Autodesk Inventor part; units mm, degrees
ref_plane "YZ-Ebene" through (0, 0, 0) normal (1, 0, 0) x (0, 1, 0)
ref_plane "XZ-Ebene" through (0, 0, 0) normal (0, 1, 0) x (-1, 0, 0)
sketch "Skizze1" plane through (0, 0, 0) normal (0, 0, 1) x (1, 0, 0)
  line L0 (-14.4, 0) -> (2.4, 0)
  line L1 (0, -0.9) -> (0, 5.4)
  line L2 (-12, 1.7) -> (-12, 2)
  line L3 (-12, 2) -> (-11, 2)
  line L4 (-11, 2) -> (-11, 4.5)
  line L5 (-11, 4.5) -> (0, 4.5)
  line L6 (-12, 1.7) -> (0, 1.7)
  line L7 (0, 4.5) -> (0, 1.7)
  point P0 (0, 0)
  dimension "d1" = 3.4
  dimension "d2" = 4
  dimension "d3" = 11
  dimension "d4" = 12
  dimension "d5" = 9
revolve "Umdrehung1" add sketch "Skizze1" angle 360 about axis through (-10, 0, 0) along (1, 0, 0)
ref_plane "Arbeitsebene1" through (-5.5, 0, 4.5) normal (0, 0, 1) x (1, 0, 0)
sketch "Skizze2" plane through (-5.5, 0, 4.5) normal (0, 0, 1) x (1, 0, 0)
  line L0 (-5.5, 4.5) -> (5.5, 4.5)
  line L1 (5.5, -4.5) -> (5.5, 4.5)
  line L2 (3, 4.5) -> (5.5, 4.5)
  line L3 (5.5, 4.5) -> (5.5, 2.6)
  line L4 (5.5, 2.6) -> (3, 2.6)
  line L5 (3, 2.6) -> (3, 4.5)
  point P0 (5.5, 0)
  dimension "d9" = 1.9
  dimension "d10" = 2.5
extrude "Extrusion1" cut sketch "Skizze2" against normal through all
ref_plane "Arbeitsebene2" through (-5.5, 0, 4.5) normal (0, 0, 1) x (1, 0, 0)
sketch "Skizze3" plane through (-5.5, 0, 4.5) normal (0, 0, 1) x (1, 0, 0)
  line L0 (-8.9, 0) -> (7.9, 0)
  line L1 (-5.5, -4.5) -> (-5.5, 4.5)
  line L2 (5.5, -4.5) -> (5.5, 2.6)
  circle A0 centre (0, 0) radius 2.25
  point P0 (5.5, 0)
  dimension "d13" = 4.5
  dimension "d14" = 5.5
extrude "Extrusion2" cut sketch "Skizze3" against normal through all
properties part number "Schließbahn_ra8846s" material "Stahl"
For this review, take the finished solid that the model builds, in its own axes (mm). A direction names the side the tool comes from. Round coordinates to 2 decimals unless told otherwise and drop trailing zeros. Write each loop counter-clockwise with the first axis right and the second up, starting at its lowest first coordinate (ties: lowest second). Pieces come first, ordered by that corner, then holes.
1) For line 1 along Z through (x, y) = (-8.1, 0); line 2 along X through (y, z) = (3.5, -1.75), list the stretches that pass through material, from the lowest coordinate up.
Answer below:
line 1: z = -4.5 to -1.7, 1.7 to 4.5
line 2: x = -11 to -2.5
2) Take a section at C-C on x = -3. Give the boundary of the cut face in (y, z), then the cut area to 3 significant figures.
Answer below:
outline: circle Ø9 at (0, 0); hole circle Ø3.4 at (0, 0)
area: 54.5 mm2
3) Take a section at A-A on y = 0. Give the boundary of the cut face in (x, z).
Answer below:
outline: (-12, -2) - (-11, -2) - (-11, -4.5) - (-7.75, -4.5) - (-7.75, -1.7) - (-12, -1.7) - close; (-12, 1.7) - (-7.75, 1.7) - (-7.75, 4.5) - (-11, 4.5) - (-11, 2) - (-12, 2) - close; (-3.25, -4.5) - (0, -4.5) - (0, -1.7) - (-3.25, -1.7) - close; (-3.25, 1.7) - (0, 1.7) - (0, 4.5) - (-3.25, 4.5) - close
4) Machinability: for faces 1 (the face through (-1, 2.6, 0)), 2 (the face through (-11, 1, -2)), 3 (the face through (-5.79, 2.23, 0.06)), which of the approach directions +Z, -Z, +X, -X, +Y, -Y give a long, thin tool a straight path to every point of the face, cutting with its end or side? Answer none if there is none.
Answer below:
face 1: +Z, -Z, +X, +Y
face 2: -X
face 3: +Z, -Z
5) Mouldability with a two-part tool opening along Y and no side actions: class faces 4 (the face through (-5.423, -4.496, 0.198)), 5 (the face through (-1.99, 1.57, -0.65)), 6 (the face through (-9.45, 1.57, -0.65)), 7 (the face through (-2.5, 3, 0)) as +Y half, -Y half, draft (parallel to the pull), parting line (faces both ways), or undercut.
Answer below:
face 4: parting line
face 5: undercut
face 6: undercut
face 7: draft
6) Insertion check: pin 1 Ø1.5 at (y, z) = (4, 0) entering from +X; pin 2 Ø3 at (x, y) = (-6, -1.5) entering from +Z; pin 3 Ø0.8 at (x, z) = (-1, 1) entering from +Y. Each pin has a flat end and moves straight along its axis. Give the tip position at first contact, or say it passes through.
Answer below:
pin 1: stops at x = -2.5
pin 2: stops at z = 4.36
pin 3: stops at y = 2.6
7) Take a section at D-D on y = 1.25. Give the boundary of the cut face in (x, z), then the cut area to 3 significant figures.
Answer below:
outline: (-12, -1.56) - (-11, -1.56) - (-11, -4.32) - (-7.37, -4.32) - (-7.37, -1.15) - (-12, -1.15) - close; (-12, 1.15) - (-7.37, 1.15) - (-7.37, 4.32) - (-11, 4.32) - (-11, 1.56) - (-12, 1.56) - close; (-3.63, -4.32) - (0, -4.32) - (0, -1.15) - (-3.63, -1.15) - close; (-3.63, 1.15) - (0, 1.15) - (0, 4.32) - (-3.63, 4.32) - close
area: 46.8 mm2
8) Take a section at B-B on z = 0. Give the boundary of the cut face in (x, y).
Answer below:
outline: (-12, -2) - (-11, -2) - (-11, -4.5) - (0, -4.5) - (0, -1.7) - (-4.03, -1.7) arc R2.25 cw to (-6.97, -1.7) - (-12, -1.7) - close; (-12, 1.7) - (-6.97, 1.7) arc R2.25 cw to (-4.03, 1.7) - (0, 1.7) - (0, 2.6) - (-2.5, 2.6) - (-2.5, 4.5) - (-11, 4.5) - (-11, 2) - (-12, 2) - close
